Geometry check sheet. Reference: the model listing, model coordinates, mm. A direction names the side the tool comes from. Give positions to 0.01 mm unless a question says otherwise; leave off trailing zeros. Loops run counter-clockwise (first coordinate to the right, second up) from the corner with the lowest first, then second, coordinate; pieces in that order, holes last.
1. Cross-section at C-C, the plane z = 7.5. Record the cut outline in (x, y).
2. Cross-section at D-D, the plane y = -7.75. Record the cut outline in (x, z) (1 decimal), plus the area to 3 significant figures.
3. Go/stop test with flat-tipped pins: pin 1 Ø3 at (x, z) = (0.5, 3) entering from -Y; pin 2 Ø2 at (x, z) = (4, 7.5) entering from -Y; pin 3 Ø3 at (y, z) = (0.5, 3.5) entering from +X; pin 4 Ø2 at (y, z) = (-4, 7) entering from -X. Record where each tip stops, or that it passes through.
4. Cross-section at B-B, the plane x = -1.5. Record the cut outline in (y, z) (1 decimal).
5. Tool access check on faces 5 (the flat face through (-0.9, -9.3, 1.588)), 6 (the flat face through (-7.992, 0, 6)), 7 (the flat face through (0, -8.122, 6)), 8 (the flat face through (0, 7.553, 6)), 9 (the flat face through (-6.405, 0, 5)). Record the directions out of +Z, -Z, +X, -X, +Y, -Y that give a thin tool (end or side, any length) a straight path to the whole face; none if there is none.
6. Release check for a two-part mould opening along X. For faces 1 (the flat face through (7.683, 0, 6)), 2 (the flat face through (0, -6.534, 5)), 3 (the cylindrical face through (-8.293, -0.16, 1.873)), 4 (the cylindrical face through (-0.031, -8.422, 1.873)) record: +X half, -X half, draft (parallel to the pull), parting line (faces both ways), or undercut.
7. Material ranges on L1, parallel to X at y = -0.5, z = 4.75; L2, parallel to Y at x = 4.25, z = 5; L3, parallel to Y at x = -0.5, z = 1.25, recorded low to high.
8. Cross-section at A-A, the plane y = 2.5. Record the cut outline in (x, z) (1 decimal).
from build123d import *

# Parameters (mm, degrees)
SKETCH1_W           = 15.675
SKETCH1_H           = 15.675
SKETCH1_W_2         = 12.5
SKETCH1_H_2         = 12.5
BOSS_EXTRUDE2_DEPTH = 9.525
SKETCH1_7_W         = 18.85
SKETCH1_7_H         = 18.85
BOSS_EXTRUDE3_DEPTH = 1.5875
SKETCH1_8_W         = 12.5
SKETCH1_8_H         = 12.5
CUT_EXTRUDE3_DEPTH  = 17.636336121
FILLET4_R           = 1


with BuildPart() as part:
    # Sketch1 → Boss-Extrude2 (new body)
    with BuildSketch(Plane.XY):
        with Locations((-0.154958678, -0.284090909)):
            Rectangle(SKETCH1_W, SKETCH1_H)
        with Locations((-0.154958678, -0.284090909)):
            Rectangle(SKETCH1_W_2, SKETCH1_H_2, mode=Mode.SUBTRACT)
    extrude(amount=BOSS_EXTRUDE2_DEPTH)

    # Sketch1<7> → Boss-Extrude3 (add)
    with BuildSketch(Plane.XY):
        with Locations((-0.154958678, -0.284090909)):
            Rectangle(SKETCH1_7_W, SKETCH1_7_H)
    extrude(amount=BOSS_EXTRUDE3_DEPTH)

    # Sketch1<8> → Cut-Extrude3 (cut, through all)
    with BuildSketch(Plane.XY):
        with Locations((-0.154958678, -0.284090909)):
            Rectangle(SKETCH1_8_W, SKETCH1_8_H)
    extrude(amount=CUT_EXTRUDE3_DEPTH, mode=Mode.SUBTRACT)

    # Fillet4
    fillet4_edges = [part.edges().sort_by_distance(p)[0] for p in [
        (7.682541322, -0.284090909, 1.5875),
        (-0.154958678, 7.553409091, 1.5875),
        (-0.154958678, -8.121590909, 1.5875),
        (-7.992458678, -0.284090909, 1.5875),
    ]]
    fillet(fillet4_edges, radius=FILLET4_R)


solid = part.part
Result:
1. outline: (-7.99, -8.12) - (7.68, -8.12) - (7.68, 7.55) - (-7.99, 7.55) - close; hole (-6.4, -6.53) - (6.1, -6.53) - (6.1, 5.97) - (-6.4, 5.97) - close
2. outline: (-9.6, 0) - (9.3, 0) - (9.3, 1.6) - (8.7, 1.6) arc R1 cw to (7.7, 2.6) - (7.7, 9.5) - (-8, 9.5) - (-8, 2.6) arc R1 cw to (-9, 1.6) - (-9.6, 1.6) - close
2. area: 155 mm2
3. pin 1: stops at y = -9.71
3. pin 2: stops at y = -8.12
3. pin 3: stops at x = 7.87
3. pin 4: stops at x = -7.99
4. outline: (-9.7, 0) - (-6.5, 0) - (-6.5, 9.5) - (-8.1, 9.5) - (-8.1, 2.6) arc R1 cw to (-9.1, 1.6) - (-9.7, 1.6) - close; (6, 0) - (9.1, 0) - (9.1, 1.6) - (8.6, 1.6) arc R1 cw to (7.6, 2.6) - (7.6, 9.5) - (6, 9.5) - close
5. face 5: +Z
5. face 6: +Z, -X, +Y, -Y
5. face 7: +Z, +X, -X, -Y
5. face 8: +Z, +X, -X, +Y
5. face 9: +Z, -Z
6. face 1: +X half
6. face 2: undercut
6. face 3: -X half
6. face 4: draft
7. L1: x = -7.99 to -6.4, 6.1 to 7.68
7. L2: y = -8.12 to -6.53, 5.97 to 7.55
7. L3: y = -9.71 to -6.53, 5.97 to 9.14
8. outline: (-9.6, 0) - (-6.4, 0) - (-6.4, 9.5) - (-8, 9.5) - (-8, 2.6) arc R1 cw to (-9, 1.6) - (-9.6, 1.6) - close; (6.1, 0) - (9.3, 0) - (9.3, 1.6) - (8.7, 1.6) arc R1 cw to (7.7, 2.6) - (7.7, 9.5) - (6.1, 9.5) - close
